Input: part model. Units: mm. Frame: model coordinates. Face numbers are marked on the shaded views. Coordinates: 2 decimals unless noted, no trailing zeros. Write each loop counter-clockwise with the first axis right and the second up, starting at its lowest first coordinate (ties: lowest second). Pieces come first, ordered by that corner, then holes. Notation, with made-up numbers: M 57,-11 L 86,-11 A29 ccw 86,15 Z; hole C 57,19 d10. An arc over 180 degrees is marked long. Use one line per item in the form item = value.
from build123d import *

# Parameters (mm, degrees)
F2_DEPTH = 4
F0_R     = 11.5
F3_DEPTH = 4


with BuildPart() as f2:
    # F1 (on Top) → F2 (new body, symmetric)
    with BuildSketch(Plane.XY):
        with BuildLine():
            ThreePointArc((-13.5999908393, -7.4780133596), (-11.983461177, -3.8932487735), (-11.43, 0))
            ThreePointArc((-11.43, 0), (-11.9830626174, 3.891875033), (-13.5984597383, 7.4755967957))
            add(Edge.make_bspline(
                [(-15.8525407314, 0), (-15.8522471897, 2.5837824299), (-15.0093024718, 5.1671341097), (-13.5984597383, 7.4755967957)],
                knots=[0, 0, 0, 0, 0.0815141474, 0.0815141474, 0.0815141474, 0.0815141474], degree=3))
            add(Edge.make_bspline(
                [(-13.5999908393, -7.4780133596), (-15.0104036313, -5.1682195796), (-15.8528342859, -2.583894396), (-15.8525407314, 0)],
                knots=[0.9184823203, 0.9184823203, 0.9184823203, 0.9184823203, 1, 1, 1, 1], degree=3))
        make_face()
        with BuildLine():
            ThreePointArc((-13.5984597383, 7.4755967957), (-11.9830626174, 3.891875033), (-11.43, 0))
            ThreePointArc((-11.43, 0), (-11.983461177, -3.8932487735), (-13.5999908393, -7.4780133596))
            add(Edge.make_bspline(
                [(-7.4785417751, -13.6003257283), (-9.9432134858, -12.0948774028), (-12.0949702136, -9.9427437558), (-13.5999908393, -7.4780133596)],
                knots=[0.8314965882, 0.8314965882, 0.8314965882, 0.8314965882, 0.9184823203, 0.9184823203, 0.9184823203, 0.9184823203], degree=3))
            ThreePointArc((-7.4785417751, -13.6003257283), (0.0002714697, -11.4300000026), (7.4790003598, -13.6006163882))
            add(Edge.make_bspline(
                [(13.6008490507, -7.4793674115), (12.0955450693, -9.9436905864), (9.9436552045, -12.0954300948), (7.4790003598, -13.6006163882)],
                knots=[0.5814918981, 0.5814918981, 0.5814918981, 0.5814918981, 0.6684682369, 0.6684682369, 0.6684682369, 0.6684682369], degree=3))
            ThreePointArc((13.6008490507, -7.4793674115), (11.4300000733, -0.0014306429), (13.5993174007, 7.4769505944))
            add(Edge.make_bspline(
                [(7.4718602429, 13.5960936758), (9.9386630737, 12.0924010227), (12.0926316746, 9.941363048), (13.5993174007, 7.4769505944)],
                knots=[0.3314005666, 0.3314005666, 0.3314005666, 0.3314005666, 0.4184264481, 0.4184264481, 0.4184264481, 0.4184264481], degree=3))
            ThreePointArc((7.4718602429, 13.5960936758), (0.0002712159, 11.4300000026), (-7.4714019113, 13.5958035648))
            add(Edge.make_bspline(
                [(-13.5984597383, 7.4755967957), (-12.0920574929, 9.9404167869), (-9.9382219246, 12.0918490046), (-7.4714019113, 13.5958035648)],
                knots=[0.0815141474, 0.0815141474, 0.0815141474, 0.0815141474, 0.168549429, 0.168549429, 0.168549429, 0.168549429], degree=3))
        make_face()
        with BuildLine():
            add(Edge.make_bspline(
                [(-15.8525407314, 0), (-15.8522471897, 2.5837824299), (-15.0093024718, 5.1671341097), (-13.5984597383, 7.4755967957)],
                knots=[0, 0, 0, 0, 0.0815141474, 0.0815141474, 0.0815141474, 0.0815141474], degree=3))
            ThreePointArc((-13.5984597383, 7.4755967957), (-39.3699999268, 0.001430389), (-13.5999908393, -7.4780133596))
            add(Edge.make_bspline(
                [(-13.5999908393, -7.4780133596), (-15.0104036313, -5.1682195796), (-15.8528342859, -2.583894396), (-15.8525407314, 0)],
                knots=[0.9184823203, 0.9184823203, 0.9184823203, 0.9184823203, 1, 1, 1, 1], degree=3))
        make_face()
        with BuildLine():
            add(Edge.make_bspline(
                [(-7.4714019113, 13.5958035648), (-5.1635862062, 15.0028174269), (-6.01624e-05, 16.6834550003), (5.1637921907, 15.0030261348), (7.4718602429, 13.5960936758)],
                knots=[0.168549429, 0.168549429, 0.168549429, 0.168549429, 0.2499746601, 0.3314005666, 0.3314005666, 0.3314005666, 0.3314005666], degree=3))
            ThreePointArc((-7.4714019113, 13.5958035648), (0.0002712159, 11.4300000026), (7.4718602429, 13.5960936758))
        make_face()
        with BuildLine():
            ThreePointArc((13.97, 25.4), (-6.7374110495, 37.6379815472), (-7.4714019113, 13.5958035648))
            add(Edge.make_bspline(
                [(-7.4714019113, 13.5958035648), (-5.1635862062, 15.0028174269), (-6.01624e-05, 16.6834550003), (5.1637921907, 15.0030261348), (7.4718602429, 13.5960936758)],
                knots=[0.168549429, 0.168549429, 0.168549429, 0.168549429, 0.2499746601, 0.3314005666, 0.3314005666, 0.3314005666, 0.3314005666], degree=3))
            ThreePointArc((7.4718602429, 13.5960936758), (12.2381123461, 18.662826542), (13.97, 25.4))
        make_face()
        with BuildLine():
            add(Edge.make_bspline(
                [(7.4790003598, -13.6006163882), (5.169117738, -15.0112819299), (-6.05056e-05, -16.6968060532), (-5.1689117665, -15.0110728934), (-7.4785417751, -13.6003257283)],
                knots=[0.6684682369, 0.6684682369, 0.6684682369, 0.6684682369, 0.7499827475, 0.8314965882, 0.8314965882, 0.8314965882, 0.8314965882], degree=3))
            ThreePointArc((-7.4785417751, -13.6003257283), (-6.7337089112, -37.6400189664), (13.97, -25.4))
            ThreePointArc((13.97, -25.4), (12.2401498158, -18.6665289421), (7.4790003598, -13.6006163882))
        make_face()
        with BuildLine():
            ThreePointArc((7.4790003598, -13.6006163882), (0.0002714697, -11.4300000026), (-7.4785417751, -13.6003257283))
            add(Edge.make_bspline(
                [(7.4790003598, -13.6006163882), (5.169117738, -15.0112819299), (-6.05056e-05, -16.6968060532), (-5.1689117665, -15.0110728934), (-7.4785417751, -13.6003257283)],
                knots=[0.6684682369, 0.6684682369, 0.6684682369, 0.6684682369, 0.7499827475, 0.8314965882, 0.8314965882, 0.8314965882, 0.8314965882], degree=3))
        make_face()
        with BuildLine():
            add(Edge.make_bspline(
                [(13.5993174007, 7.4769505944), (15.010869159, 5.1681441381), (16.697763129, 0.000319146), (15.0119706471, -5.1692295952), (13.6008490507, -7.4793674115)],
                knots=[0.4184264481, 0.4184264481, 0.4184264481, 0.4184264481, 0.4999574097, 0.5814918981, 0.5814918981, 0.5814918981, 0.5814918981], degree=3))
            ThreePointArc((13.5993174007, 7.4769505944), (11.4300000733, -0.0014306429), (13.6008490507, -7.4793674115))
        make_face()
        with BuildLine():
            ThreePointArc((39.37, 0), (29.292644608, 13.4167141266), (13.5993174007, 7.4769505944))
            add(Edge.make_bspline(
                [(13.5993174007, 7.4769505944), (15.010869159, 5.1681441381), (16.697763129, 0.000319146), (15.0119706471, -5.1692295952), (13.6008490507, -7.4793674115)],
                knots=[0.4184264481, 0.4184264481, 0.4184264481, 0.4184264481, 0.4999574097, 0.5814918981, 0.5814918981, 0.5814918981, 0.5814918981], degree=3))
            ThreePointArc((13.6008490507, -7.4793674115), (29.2940185695, -13.4163154175), (39.37, 0))
        make_face()
    extrude(amount=F2_DEPTH, both=True)

    # F0 (on Top) → F3 (cut, symmetric)
    with BuildSketch(Plane.XY):
        Circle(F0_R)
        with Locations((0, -25.4)):
            Circle(F0_R)
        with Locations((25.4, 0)):
            Circle(F0_R)
        with Locations((0, 25.4)):
            Circle(F0_R)
        with Locations((-25.4, 0)):
            Circle(F0_R)
    extrude(amount=F3_DEPTH, both=True, mode=Mode.SUBTRACT)


solid = f2.part
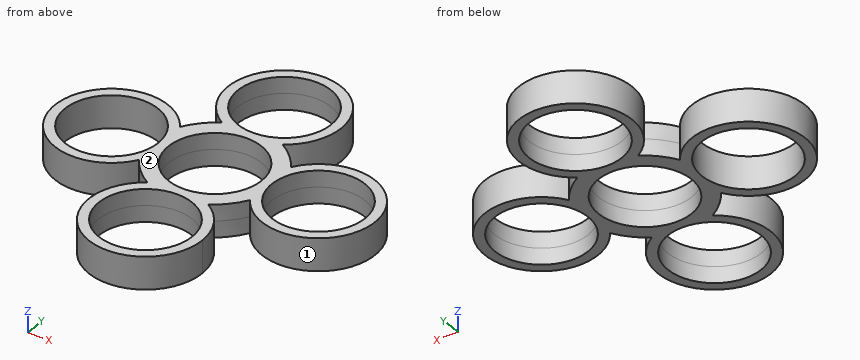
(1) Section query D-D on y = 30.5. Return the cut outline in (x, z).
Computed:
outline = M -13.01,-4 L -10.31,-4 L -10.31,4 L -13.01,4 Z; M 10.31,-4 L 13.01,-4 L 13.01,4 L 10.31,4 Z
(2) First-contact query: pin 1 Ø4 at (y, z) = (22, -0.5) entering from +X; pin 2 Ø3 at (x, z) = (-17.5, -2.5) entering from -Y; pin 3 Ø3 at (x, z) = (27.5, 3) entering from +Y. Flat tips, straight axial feed; report the tip coordinate or a pass-through.
Computed:
pin_1 = 13.9
pin_2 = -12.42
pin_3 = 13.96
(3) Pull-direction query (X, two-part tool) for the marked faces 1 and 2; classes: pulls with the +X half, pulls with the -X half, needs draft (parallel to the pull), parting line crosses it, or undercut.
Computed:
face_1 = undercut
face_2 = needs draft
(4) Section query C-C on x = 25.4. Return the cut outline in (y, z), plus the area to 3 significant figures.
Computed:
outline = M -13.97,-4 L -11.5,-4 L -11.5,4 L -13.97,4 Z; M 11.5,-4 L 13.97,-4 L 13.97,4 L 11.5,4 Z
area = 39.5 mm^2
(5) Section query A-A on y = 0. Return the cut outline in (x, z).
Computed:
outline = M -39.37,-4 L -36.9,-4 L -36.9,4 L -39.37,4 Z; M -13.9,-4 L -11.5,-4 L -11.5,4 L -13.9,4 Z; M 11.5,-4 L 13.9,-4 L 13.9,4 L 11.5,4 Z; M 36.9,-4 L 39.37,-4 L 39.37,4 L 36.9,4 Z
(6) Line query: probe 1 along Y at (x, z) = (0, -2); probe 2 along Y at (x, z) = (25.4, -1.05). Output: solid intervals per line, ascending.
Computed:
probe_1 = -39.37 to -36.9, -13.9 to -11.5, 11.5 to 13.9, 36.9 to 39.37
probe_2 = -13.97 to -11.5, 11.5 to 13.97
